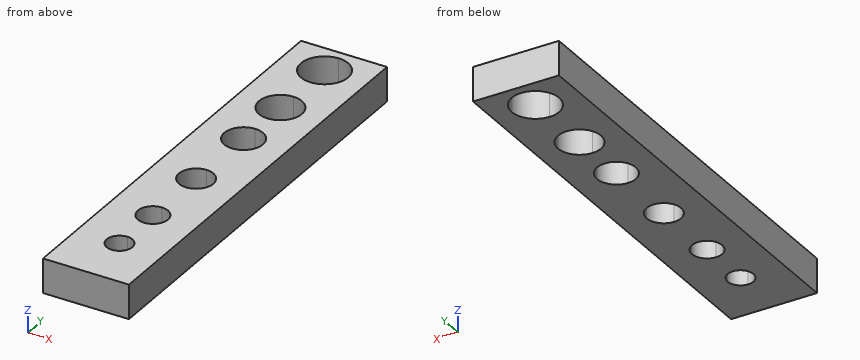
```python
from build123d import *

# Parameters (mm, degrees)
F0_W     = 10
F0_H     = 50
F1_DEPTH = 4
F3_DEPTH = 4.001


with BuildPart() as f1:
    # F0 (on Top) → F1 (new body)
    with BuildSketch(Plane.XY):
        with Locations((5, 25)):
            Rectangle(F0_W, F0_H)
    extrude(amount=F1_DEPTH)

    # F2 (on face) → F3 (cut, through all)
    with BuildSketch(Plane.XY.offset(4)):
        with BuildLine():
            ThreePointArc((5, 5), (6.06066, 5.43934), (6.5, 6.5))
            ThreePointArc((6.5, 6.5), (6.06066, 7.56066), (5, 8))
            Line((5, 8), (5, 5))
        make_face()
        with BuildLine():
            ThreePointArc((5, 48.97335), (2.25, 46.22335), (5, 43.47335))
            Line((5, 43.47335), (5, 48.97335))
        make_face()
        with BuildLine():
            Line((5, 48.97335), (5, 43.47335))
            ThreePointArc((5, 43.47335), (6.944544, 44.278806), (7.75, 46.22335))
            ThreePointArc((7.75, 46.22335), (6.944544, 48.167894), (5, 48.97335))
        make_face()
        with BuildLine():
            ThreePointArc((5, 40.173719), (2.5, 37.673719), (5, 35.173719))
            Line((5, 35.173719), (5, 40.173719))
        make_face()
        with BuildLine():
            Line((5, 40.173719), (5, 35.173719))
            ThreePointArc((5, 35.173719), (6.767767, 35.905952), (7.5, 37.673719))
            ThreePointArc((7.5, 37.673719), (6.767767, 39.441486), (5, 40.173719))
        make_face()
        with BuildLine():
            ThreePointArc((5, 32.784836), (2.75, 30.534836), (5, 28.284836))
            Line((5, 28.284836), (5, 32.784836))
        make_face()
        with BuildLine():
            Line((5, 32.784836), (5, 28.284836))
            ThreePointArc((5, 28.284836), (6.59099, 28.943845), (7.25, 30.534836))
            ThreePointArc((7.25, 30.534836), (6.59099, 32.125826), (5, 32.784836))
        make_face()
        with BuildLine():
            ThreePointArc((5, 23.35), (3, 21.35), (5, 19.35))
            Line((5, 19.35), (5, 23.35))
        make_face()
        with BuildLine():
            Line((5, 23.35), (5, 19.35))
            ThreePointArc((5, 19.35), (6.414214, 19.935786), (7, 21.35))
            ThreePointArc((7, 21.35), (6.414214, 22.764214), (5, 23.35))
        make_face()
        with BuildLine():
            ThreePointArc((5, 14.724094), (3.25, 12.974094), (5, 11.224094))
            Line((5, 11.224094), (5, 14.724094))
        make_face()
        with BuildLine():
            Line((5, 14.724094), (5, 11.224094))
            ThreePointArc((5, 11.224094), (6.237437, 11.736657), (6.75, 12.974094))
            ThreePointArc((6.75, 12.974094), (6.237437, 14.211531), (5, 14.724094))
        make_face()
        with BuildLine():
            Line((5, 5), (5, 8))
            ThreePointArc((5, 8), (3.5, 6.5), (5, 5))
        make_face()
    extrude(amount=-F3_DEPTH, mode=Mode.SUBTRACT)


solid = f1.part
```
Geometry: final body of the model. Coordinates: model frame, mm. Round coordinates to 2 decimals unless told otherwise and drop trailing zeros. Write each loop counter-clockwise with the first axis right and the second up, starting at its lowest first coordinate (ties: lowest second). Pieces come first, ordered by that corner, then holes.
Item 1: Section query C-C (y = 44). Return loops of the section in (x, z).
Item 2: Section query B-B (z = 1.7). Return loops of the section in (x, y).
Item 3: Pin query (flat end, axial travel): P1, Ø1, axis at x = 6, y = 20, coming from the +Z side. Return the tip coordinate at first contact, or that it passes through.
Item 4: Material intervals for L1, parallel to X at y = 47.5, z = 2.3; L2, parallel to X at y = 14.5, z = 0.95, sorted ascending.
Item 5: Section query A-A (y = 12). Return loops of the section in (x, z), plus the area to 3 significant figures.
Completed:
1. outline: (0, 0) - (3.38, 0) - (3.38, 4) - (0, 4) - close; (6.62, 0) - (10, 0) - (10, 4) - (6.62, 4) - close
2. outline: (0, 0) - (10, 0) - (10, 50) - (0, 50) - close; hole circle Ø5 at (5, 37.67); hole circle Ø3.5 at (5, 12.97); hole (5, 8) arc R1.5 ccw (long way) to (6.5, 6.5) arc R1.5 ccw to start; hole (5, 19.35) arc R2 ccw to (7, 21.35) arc R2 ccw to (5, 23.35) arc R2 ccw to start; hole (5, 32.78) arc R2.25 ccw (long way) to (7.25, 30.53) arc R2.25 ccw to start; hole (5, 43.47) arc R2.75 ccw to (7.75, 46.22) arc R2.75 ccw to (5, 48.97) arc R2.75 ccw to start
3. P1: stops at z = 4
4. L1: x = 0 to 2.56, 7.44 to 10
4. L2: x = 0 to 4.14, 5.86 to 10
5. outline: (0, 0) - (3.55, 0) - (3.55, 4) - (0, 4) - close; (6.45, 0) - (10, 0) - (10, 4) - (6.45, 4) - close
5. area: 28.4 mm2
